The listing builds one solid part. Answer for the finished solid, in the listing's coordinates (mm). A direction names the side the tool comes from. Give positions to 0.01 mm unless a question says otherwise; leave off trailing zeros. Order: outer loops, then holes, each group sorted by start corner. A loop starts at its lowest first (then second) coordinate and runs counter-clockwise, first axis right, second up. Notation, with made-up numbers: (-32.5, 34.25) - (-23.5, 34.25) arc R26 ccw to (-23.5, 52.25) - close; hole circle Ø2 at (-30.5, -14). An arc over 180 degrees is marked (long way). Answer in a Markdown table with one row per item.
from build123d import *

# Parameters (mm, degrees)
SKETCH1_W                            = 110
SKETCH1_H                            = 75
BOSS_EXTRUDE1_DEPTH                  = 6
SKETCH2_W                            = 90
SKETCH2_H                            = 18
CUT_EXTRUDE1_DEPTH                   = 10
FILLET1_R                            = 3
F_3_9_3_9_DIAMETER_HOLE1_D           = 3.9
F_3_9_3_9_DIAMETER_HOLE1_DEPTH       = 15
F_3_9_3_9_DIAMETER_HOLE1_CSINK_D     = 3.95
F_3_9_3_9_DIAMETER_HOLE1_CSINK_ANGLE = 90
F_3_9_3_9_DIAMETER_HOLE1_TIP         = 1.171678207
FILLET2_R                            = 3
SKETCH6_R                            = 7.5
BOSS_EXTRUDE3_DEPTH                  = 10
SKETCH7_R                            = 4
CUT_EXTRUDE2_DEPTH                   = 3.5


with BuildPart() as part:
    # Sketch1 → Boss-Extrude1 (new body)
    with BuildSketch(Plane(origin=(0, 0, 0), x_dir=(1, 0, 0), z_dir=(0, 1, 0))):
        Rectangle(SKETCH1_W, SKETCH1_H)
    extrude(amount=BOSS_EXTRUDE1_DEPTH)

    # Sketch2 → Cut-Extrude1 (cut)
    with BuildSketch(Plane(origin=(0, 6, 0), x_dir=(1, 0, 0), z_dir=(0, 1, 0))):
        Rectangle(SKETCH2_W, SKETCH2_H)
    extrude(amount=-CUT_EXTRUDE1_DEPTH, mode=Mode.SUBTRACT)

    # Fillet1
    fillet1_edges = [part.edges().sort_by_distance(p)[0] for p in [
        (45, 3, -9),
        (45, 3, 9),
        (-45, 3, 9),
        (-45, 3, -9),
    ]]
    fillet(fillet1_edges, radius=FILLET1_R)

    # Ø3.9 (3.9) Diameter Hole1
    with Locations(Plane(origin=(0, 0, 0), x_dir=(-1, 0, 0), z_dir=(0, -1, 0))):
        with Locations((0, 0), (8.25, -12.5), (-8.25, 12.5), (-8.25, -12.5), (8.25, 12.5), (24.75, -12.5), (41.25, -12.5), (24.75, 12.5), (41.25, 12.5), (-24.75, 12.5), (-41.25, 12.5), (-24.75, -12.5), (-41.25, -12.5)):
            CounterSinkHole(F_3_9_3_9_DIAMETER_HOLE1_D / 2, F_3_9_3_9_DIAMETER_HOLE1_CSINK_D / 2, depth=F_3_9_3_9_DIAMETER_HOLE1_DEPTH, counter_sink_angle=F_3_9_3_9_DIAMETER_HOLE1_CSINK_ANGLE)
            with Locations((0, 0, -(F_3_9_3_9_DIAMETER_HOLE1_DEPTH + F_3_9_3_9_DIAMETER_HOLE1_TIP / 2))):  # 118° drill point
                Cone(0, F_3_9_3_9_DIAMETER_HOLE1_D / 2, F_3_9_3_9_DIAMETER_HOLE1_TIP, mode=Mode.SUBTRACT)

    # Fillet2
    fillet2_edges = [part.edges().sort_by_distance(p)[0] for p in [
        (55, 3, 37.5),
        (-55, 3, 37.5),
        (-55, 3, -37.5),
        (55, 3, -37.5),
    ]]
    fillet(fillet2_edges, radius=FILLET2_R)

    # Sketch6 → Boss-Extrude3 (add)
    with BuildSketch(Plane(origin=(0, 6, 0), x_dir=(1, 0, 0), z_dir=(0, 1, 0))):
        with Locations(Location((-30, -30, 0), (0, 0, 270))):
            Circle(SKETCH6_R)
        with Locations(Location((30, -30, 0), (0, 0, 270))):
            Circle(SKETCH6_R)
        with Locations(Location((30, 30, 0), (0, 0, 90))):
            Circle(SKETCH6_R)
        with Locations(Location((-30, 30, 0), (0, 0, 90))):
            Circle(SKETCH6_R)
    extrude(amount=BOSS_EXTRUDE3_DEPTH)

    # Sketch7 → Cut-Extrude2 (cut)
    with BuildSketch(Plane(origin=(0, 16, 0), x_dir=(1, 0, 0), z_dir=(0, 1, 0))):
        with Locations(Location((-30, 30, 0), (0, 0, 270))):
            Circle(SKETCH7_R)
        with Locations(Location((30, 30, 0), (0, 0, 270))):
            Circle(SKETCH7_R)
        with Locations(Location((30, -30, 0), (0, 0, 270))):
            Circle(SKETCH7_R)
        with Locations(Location((-30, -30, 0), (0, 0, 270))):
            Circle(SKETCH7_R)
    extrude(amount=-CUT_EXTRUDE2_DEPTH, mode=Mode.SUBTRACT)


solid = part.part
Item 1: Find section C-C on z = -2.5. Write down the section's boundary in (x, y), then the cut area to 3 significant figures.
Answer block:
| item | result |
|---|---|
| outline | (-55, 0) - (-45, 0) - (-45, 6) - (-55, 6) - close; (45, 0) - (55, 0) - (55, 6) - (45, 6) - close |
| area | 120 mm² |
Item 2: Each of these flat-tipped pins is pushed along its axis until it touches: P1, Ø7, axis at x = -30, z = -30, coming from the +Y side; P2, Ø5, axis at x = 8.25, z = -12.5, coming from the +Y side; P3, Ø7, axis at x = -30, z = 30, coming from the -Y side; P4, Ø1.5, axis at x = -12, y = 8, coming from the -Z side. Where does it stop, or does it pass through?
Answer block:
| item | result |
|---|---|
| P1 | y = 12.5 |
| P2 | y = 6 |
| P3 | y = 0 |
| P4 | through |
Item 3: Find section A-A on x = -14. Write down the section's boundary in (y, z).
Answer block:
| item | result |
|---|---|
| outline | (0, -37.5) - (6, -37.5) - (6, -9) - (0, -9) - close; (0, 9) - (6, 9) - (6, 37.5) - (0, 37.5) - close |
Item 4: Determine the mould class of faces 1 (the face through (43.05, 3.05, 13.25)), 2 (the face through (-1, 0, 16)), 3 (the face through (-55, 3, 0)) for opening direction X: pulls with the +X half, pulls with the -X half, needs draft (parallel to the pull), parting line crosses it, or undercut.
Answer block:
| item | result |
|---|---|
| face 1 | undercut |
| face 2 | needs draft |
| face 3 | pulls with the -X half |
Item 5: Find section D-D on y = 9. Write down the section's boundary in (x, z), then the cut area to 3 significant figures.
Answer block:
| item | result |
|---|---|
| outline | circle Ø15 at (-30, -30); circle Ø15 at (-30, 30); circle Ø15 at (30, -30); circle Ø15 at (30, 30) |
| area | 707 mm² |
Item 6: Find section B-B on y = 4.25. Count the separate pieces of the cut face and the enclosed holes in it, then the cut area to 3 significant figures.
Answer block:
| item | result |
|---|---|
| separate pieces | 1 |
| enclosed holes | 13 |
| area | 6,490 mm² |
Item 7: Which of the six approach directions +Z, -Z, +X, -X, +Y, -Y give full straight-line access (tool end or side, diameter ignored) to faces 4 (the face through (-1, 3, -9)), 5 (the face through (-30, 12.5, -30))?
Answer block:
| item | result |
|---|---|
| face 4 | +Y, -Y |
| face 5 | +Y |
Item 8: Consider line 1 (Z direction, x = 41.25, y = 1.5); line 2 (Z direction, x = -20.5, y = 1.75); line 3 (Y direction, x = -22.5, z = 34). Determine where each line is inside the solid, lowest interval first.
Answer block:
| item | result |
|---|---|
| line 1 | -37.5 to -14.45, -10.55 to -9, 9 to 10.55, 14.45 to 37.5 |
| line 2 | -37.5 to -9, 9 to 37.5 |
| line 3 | 0 to 6 |
